from build123d import *
from build123d.topology import SkipClean

# Parameters (mm, degrees)
SKETCH1_W                = 100
SKETCH1_H                = 140
SKETCH1_R                = 2
EXTRUDE1_DEPTH           = 2
SKETCH2_W                = 60
SKETCH2_H                = 50
EXTRUDE2_DEPTH           = 87.046499057
SKETCH3_W                = 40
SKETCH3_H                = 20
EXTRUDE3_DEPTH           = 87.046499057
FILLET1_R                = 3
SKETCH4_W                = 6
SKETCH4_H                = 8
EXTRUDE4_DEPTH           = 60
SKETCH5_R                = 1
EXTRUDE5_DEPTH           = 8
SKETCH6_R                = 2
SKETCH6_R_2              = 2.1
EXTRUDE6_DEPTH           = 10
EXTRUDE_START            = -3
SKETCH_3_R               = 1.5
EXTRUDE_1_DEPTH          = 3
CUT_EXTRUDE_3_DEPTH      = 29
CUT_EXTRUDE_3_DEPTH_BACK = 134
SKETCH_4_W               = 103.957976386
SKETCH_4_H               = 74.150098407
SKETCH_6_R               = 2
CUT_EXTRUDE_4_DEPTH      = 11
SKETCH_8_R               = 2
CUT_EXTRUDE_6_DEPTH      = 11
EXTRUDE_START_2          = 1
SKETCH_9_R               = 2
SKETCH_9_R_2             = 2.1
EXTRUDE_2_DEPTH          = 1
SKETCH_10_R              = 1.6
CUT_EXTRUDE_7_DEPTH      = 3


with BuildPart() as part:
    # Sketch1 → Extrude1 (new body)
    with BuildSketch(Plane(origin=(0, 0, 0), x_dir=(1, 0, 0), z_dir=(0, 1, 0))):
        Rectangle(SKETCH1_W, SKETCH1_H)
        with Locations(Location((45, 65, 0), (0, 0, 270))):
            Circle(SKETCH1_R, mode=Mode.SUBTRACT)
        with Locations(Location((-45, 65, 0), (0, 0, 90))):
            Circle(SKETCH1_R, mode=Mode.SUBTRACT)
        with Locations(Location((-45, -65, 0), (0, 0, 270))):
            Circle(SKETCH1_R, mode=Mode.SUBTRACT)
        with Locations(Location((45, -65, 0), (0, 0, 90))):
            Circle(SKETCH1_R, mode=Mode.SUBTRACT)
    extrude(amount=EXTRUDE1_DEPTH)

    # Sketch2 → Extrude2 (cut, through all)
    with BuildSketch(Plane(origin=(0, 2, 0), x_dir=(1, 0, 0), z_dir=(0, 1, 0))):
        with Locations((0, -30)):
            Rectangle(SKETCH2_W, SKETCH2_H)
    extrude(amount=-EXTRUDE2_DEPTH, mode=Mode.SUBTRACT)

    # Sketch3 → Extrude3 (cut, through all)
    with BuildSketch(Plane(origin=(0, 2, 0), x_dir=(1, 0, 0), z_dir=(0, 1, 0))):
        with Locations((0, 30)):
            Rectangle(SKETCH3_W, SKETCH3_H)
    extrude(amount=-EXTRUDE3_DEPTH, mode=Mode.SUBTRACT)

    # Fillet1
    fillet1_edges = [part.edges().sort_by_distance(p)[0] for p in [
        (30, 1, 5),
        (30, 1, 55),
        (-30, 1, 55),
        (-30, 1, 5),
        (-20, 1, -20),
        (-20, 1, -40),
        (20, 1, -40),
        (20, 1, -20),
        (50, 1, 70),
        (-50, 1, 70),
        (-50, 1, -70),
        (50, 1, -70),
    ]]
    fillet(fillet1_edges, radius=FILLET1_R)

    # Sketch4 → Extrude4 (add)
    with BuildSketch(Plane.XZ):
        with Locations((47, 44)):
            Rectangle(SKETCH4_W, SKETCH4_H)
        with Locations((47, -24)):
            Rectangle(SKETCH4_W, SKETCH4_H)
        with Locations((-47, -24)):
            Rectangle(SKETCH4_W, SKETCH4_H)
        with Locations((-47, 44)):
            Rectangle(SKETCH4_W, SKETCH4_H)
    extrude(amount=EXTRUDE4_DEPTH)

    # Sketch5 → Extrude5 (add)
    # profile 1 of 4: a face of its own
    with BuildSketch(Plane.XZ.offset(60)):
        with BuildLine():
            Line((44, 40), (44, 48))
            Line((44, 48), (54, 48))
            ThreePointArc((54, 48), (58, 44), (54, 40))
            Line((54, 40), (44, 40))
        make_face()
        with Locations(Location((54, 44, 0), (0, 0, 270))):
            Circle(SKETCH5_R, mode=Mode.SUBTRACT)
    # profile 2 of 4: a face of its own
    with BuildSketch(Plane.XZ.offset(60)):
        with BuildLine():
            Line((44, -28), (44, -20))
            Line((44, -20), (54, -20))
            ThreePointArc((54, -20), (58, -24), (54, -28))
            Line((54, -28), (44, -28))
        make_face()
        with Locations(Location((54, -24, 0), (0, 0, 270))):
            Circle(SKETCH5_R, mode=Mode.SUBTRACT)
    # profile 3 of 4: a face of its own
    with BuildSketch(Plane.XZ.offset(60)):
        with BuildLine():
            Line((-44, -20), (-54, -20))
            ThreePointArc((-54, -20), (-58, -24), (-54, -28))
            Line((-54, -28), (-44, -28))
            Line((-44, -28), (-44, -20))
        make_face()
        with Locations(Location((-54, -24, 0), (0, 0, 90))):
            Circle(SKETCH5_R, mode=Mode.SUBTRACT)
    # profile 4 of 4: a face of its own
    with BuildSketch(Plane.XZ.offset(60)):
        with BuildLine():
            Line((-44, 48), (-54, 48))
            ThreePointArc((-54, 48), (-58, 44), (-54, 40))
            Line((-54, 40), (-44, 40))
            Line((-44, 40), (-44, 48))
        make_face()
        with Locations(Location((-54, 44, 0), (0, 0, 90))):
            Circle(SKETCH5_R, mode=Mode.SUBTRACT)
    extrude(amount=-EXTRUDE5_DEPTH)

    # Sketch6 → Extrude6 (cut)
    with BuildSketch(Plane(origin=(0, 0, 0), x_dir=(-1, 0, 0), z_dir=(0, -1, 0))):
        with Locations(Location((-47, -44, 0), (0, 0, 90))):
            Circle(SKETCH6_R)
        with Locations(Location((-47, 40, 0), (0, 0, 90))):
            Circle(SKETCH6_R_2)
        with Locations(Location((47, 40, 0), (0, 0, 270))):
            Circle(SKETCH6_R_2)
        with Locations(Location((47, -44, 0), (0, 0, 270))):
            Circle(SKETCH6_R)
    extrude(amount=-EXTRUDE6_DEPTH, mode=Mode.SUBTRACT)

    # Sketch 3 → Extrude 1 (add)
    # profile 1 of 4: a face of its own
    with BuildSketch(Plane(origin=(0, 2, 0), x_dir=(1, 0, 0), z_dir=(0, 1, 0)).offset(EXTRUDE_START)):
        with BuildLine():
            Line((50, 28), (50, 20))
            Line((50, 20), (54, 20))
            ThreePointArc((54, 20), (58, 24), (54, 28))
            Line((54, 28), (50, 28))
        make_face()
        with Locations(Location((54, 24, 0), (0, 0, 270))):
            Circle(SKETCH_3_R, mode=Mode.SUBTRACT)
    # profile 2 of 4: a face of its own
    with BuildSketch(Plane(origin=(0, 2, 0), x_dir=(1, 0, 0), z_dir=(0, 1, 0)).offset(EXTRUDE_START)):
        with BuildLine():
            Line((50, -40), (50, -48))
            Line((50, -48), (54, -48))
            ThreePointArc((54, -48), (58, -44), (54, -40))
            Line((54, -40), (50, -40))
        make_face()
        with Locations(Location((54, -44, 0), (0, 0, 270))):
            Circle(SKETCH_3_R, mode=Mode.SUBTRACT)
    # profile 3 of 4: a face of its own
    with BuildSketch(Plane(origin=(0, 2, 0), x_dir=(1, 0, 0), z_dir=(0, 1, 0)).offset(EXTRUDE_START)):
        with BuildLine():
            Line((-54, -48), (-50, -48))
            Line((-50, -48), (-50, -40))
            Line((-50, -40), (-54, -40))
            ThreePointArc((-54, -40), (-58, -44), (-54, -48))
        make_face()
        with Locations(Location((-54, -44, 0), (0, 0, 270))):
            Circle(SKETCH_3_R, mode=Mode.SUBTRACT)
    # profile 4 of 4: a face of its own
    with BuildSketch(Plane(origin=(0, 2, 0), x_dir=(1, 0, 0), z_dir=(0, 1, 0)).offset(EXTRUDE_START)):
        with BuildLine():
            Line((-50, 20), (-50, 28))
            Line((-50, 28), (-54, 28))
            ThreePointArc((-54, 28), (-58, 24), (-54, 20))
            Line((-54, 20), (-50, 20))
        make_face()
        with Locations(Location((-54, 24, 0), (0, 0, 270))):
            Circle(SKETCH_3_R, mode=Mode.SUBTRACT)
    extrude(amount=EXTRUDE_1_DEPTH)

    # Sketch 4 → Cut-Extrude 3 (cut, two sides: drawn at the far end of the back side and taken through both)
    with BuildSketch(Plane(origin=(50, 0, 0), x_dir=(0, 0, -1), z_dir=(1, 0, 0)).offset(-CUT_EXTRUDE_3_DEPTH_BACK)):
        with Locations((3.978988193, -38.075049204)):
            Rectangle(SKETCH_4_W, SKETCH_4_H)
    extrude(amount=CUT_EXTRUDE_3_DEPTH + CUT_EXTRUDE_3_DEPTH_BACK, mode=Mode.SUBTRACT)

    # Sketch 6 → Cut-Extrude 4 (cut)
    with BuildSketch(Plane(origin=(0, 2, 0), x_dir=(1, 0, 0), z_dir=(0, 1, 0))):
        with Locations(Location((-25, 60.55, 0), (0, 0, 270))):
            Circle(SKETCH_6_R)
        with Locations(Location((25, 60.55, 0), (0, 0, 270))):
            Circle(SKETCH_6_R)
    extrude(amount=-CUT_EXTRUDE_4_DEPTH, mode=Mode.SUBTRACT)

    # Sketch 8 → Cut-Extrude 6 (cut)
    with BuildSketch(Plane(origin=(0, 0, 0), x_dir=(-1, 0, 0), z_dir=(0, -1, 0))):
        with Locations(Location((25, -62.44, 0), (0, 0, 90))):
            Circle(SKETCH_8_R)
        with Locations(Location((-25, -62.44, 0), (0, 0, 270))):
            Circle(SKETCH_8_R)
    extrude(amount=-CUT_EXTRUDE_6_DEPTH, mode=Mode.SUBTRACT)

    # Sketch 9 → Extrude 2 (add)
    with BuildSketch(Plane.XZ.offset(EXTRUDE_START_2)):
        with BuildLine():
            Line((-44, 40), (-50, 40))
            Line((-50, 40), (-50, -20))
            Line((-50, -20), (-44, -20))
            Line((-44, -20), (-44, -28))
            Line((-44, -28), (-50, -28))
            Line((-50, -28), (-50, -67))
            ThreePointArc((-50, -67), (-49.121320344, -69.121320344), (-47, -70))
            Line((-47, -70), (47, -70))
            ThreePointArc((47, -70), (49.121320344, -69.121320344), (50, -67))
            Line((50, -67), (50, -28))
            Line((50, -28), (44, -28))
            Line((44, -28), (44, -20))
            Line((44, -20), (50, -20))
            Line((50, -20), (50, 40))
            Line((50, 40), (44, 40))
            Line((44, 40), (44, 48))
            Line((44, 48), (50, 48))
            Line((50, 48), (50, 67))
            ThreePointArc((50, 67), (49.121320344, 69.121320344), (47, 70))
            Line((47, 70), (-47, 70))
            ThreePointArc((-47, 70), (-49.121320344, 69.121320344), (-50, 67))
            Line((-50, 67), (-50, 48))
            Line((-50, 48), (-44, 48))
            Line((-44, 48), (-44, 40))
        make_face()
        with Locations(Location((-45, 65, 0), (0, 0, 270))):
            Circle(SKETCH_9_R, mode=Mode.SUBTRACT)
        with Locations(Location((-25, 62.44, 0), (0, 0, 270))):
            Circle(SKETCH_9_R, mode=Mode.SUBTRACT)
        with Locations(Location((45, 65, 0), (0, 0, 270))):
            Circle(SKETCH_9_R, mode=Mode.SUBTRACT)
        with Locations(Location((25, 62.44, 0), (0, 0, 270))):
            Circle(SKETCH_9_R, mode=Mode.SUBTRACT)
        with Locations(Location((47, -40, 0), (0, 0, 270))):
            Circle(SKETCH_9_R_2, mode=Mode.SUBTRACT)
        with Locations(Location((45, -65, 0), (0, 0, 270))):
            Circle(SKETCH_9_R, mode=Mode.SUBTRACT)
        with Locations(Location((25, -60.55, 0), (0, 0, 270))):
            Circle(SKETCH_9_R, mode=Mode.SUBTRACT)
        with Locations(Location((-45, -65, 0), (0, 0, 270))):
            Circle(SKETCH_9_R, mode=Mode.SUBTRACT)
        with Locations(Location((-47, -40, 0), (0, 0, 270))):
            Circle(SKETCH_9_R_2, mode=Mode.SUBTRACT)
        with Locations(Location((-25, -60.55, 0), (0, 0, 90))):
            Circle(SKETCH_9_R, mode=Mode.SUBTRACT)
        with BuildLine():
            Line((30, 52), (30, 8))
            ThreePointArc((30, 8), (29.121320344, 5.878679656), (27, 5))
            Line((27, 5), (-27, 5))
            ThreePointArc((-27, 5), (-29.121320344, 5.878679656), (-30, 8))
            Line((-30, 8), (-30, 52))
            ThreePointArc((-30, 52), (-29.121320344, 54.121320344), (-27, 55))
            Line((-27, 55), (27, 55))
            ThreePointArc((27, 55), (29.121320344, 54.121320344), (30, 52))
        make_face(mode=Mode.SUBTRACT)
        with BuildLine():
            Line((20, -23), (20, -37))
            ThreePointArc((20, -37), (19.121320344, -39.121320344), (17, -40))
            Line((17, -40), (-17, -40))
            ThreePointArc((-17, -40), (-19.121320344, -39.121320344), (-20, -37))
            Line((-20, -37), (-20, -23))
            ThreePointArc((-20, -23), (-19.121320344, -20.878679656), (-17, -20))
            Line((-17, -20), (17, -20))
            ThreePointArc((17, -20), (19.121320344, -20.878679656), (20, -23))
        make_face(mode=Mode.SUBTRACT)
    extrude(amount=-EXTRUDE_2_DEPTH)

    # Sketch 10 → Cut-Extrude 7 (cut)
    with SkipClean():  # the faces are left unmerged after this step: merging them gives an invalid solid
        with BuildSketch(Plane(origin=(0, -1, 0), x_dir=(-1, 0, 0), z_dir=(0, -1, 0))):
            with Locations(Location((34.25, 6.5, 0), (0, 0, 90))):
                Circle(SKETCH_10_R)
            with Locations(Location((-34.25, 6.5, 0), (0, 0, 270))):
                Circle(SKETCH_10_R)
        extrude(amount=-CUT_EXTRUDE_7_DEPTH, mode=Mode.SUBTRACT)
    add(part.part.scale(1), mode=Mode.REPLACE)  # the faces are merged on a copy


solid = part.part
Here's how the part is built. I have some questions about the finished solid (model axes, mm). A direction names the side the tool comes from. Give positions to 0.01 mm unless a question says otherwise; leave off trailing zeros. Order: outer loops, then holes, each group sorted by start corner. A loop starts at its lowest first (then second) coordinate and runs counter-clockwise, first axis right, second up. Notation, with made-up numbers: M -21,-27.75 L 13,-27.75 A21 ccw 13,-4.75 Z; hole C 67,-37.75 d10. An arc over 180 degrees is marked long. Answer as a JSON object with one key per item and string values. Group by question number.
1) Suppose I cut it at B-B, the plane z = 11.5. Write out the boundary of the cut face in (x, y).
2) We'd pull the mould along Z, two halves only. Please class faces 1 (the flat face through (50, 0, -48)), 2 (the cylindrical face through (-54.9, 0.5, 42.8)), 3 (the flat face through (-50, 0, 10)), 4 (the flat face through (1, 0, 70)): pulls with the +Z half, pulls with the -Z half, needs draft (parallel to the pull), parting line crosses it, or undercut.
3) Please list where these lines run through material, in increasing order: L1, parallel to X at y = 0.85, z = -60.55; L2, parallel to X at y = 1.45, z = 44; L3, parallel to Z at x = -6.5, y = 0.25. Write a range as [from, to].
4) Suppose I cut it at A-A, the plane x = 34.25. Write out the boundary of the cut face in (y, z), plus the area to 3 significant figures.
5) Suppose I cut it at C-C, the plane z = 44. Write out the boundary of the cut face in (x, y).
6) Suppose I cut it at D-D, the plane x = -25. Write out the boundary of the cut face in (y, z).
7) On a 3-axis mill with a long thin cutter (end or side, diameter ignored), from which of +Z, -Z, +X, -X, +Y, -Y can I reach the whole of each face in a straight line? I mean faces 5 (the cylindrical face through (45, 1, 44)), 6 (the flat face through (52, 0, -20)), 7 (the flat face through (-50, 0, -47)), 8 (the flat face through (50, 0, 57)). Say none if no direction works.
8) I'm going to push flat-ended pins straight in: pin 1 Ø2 at (x, z) = (24, 53.5) entering from -Y (3 decimals); pin 2 Ø1.1 at (y, z) = (-0.5, 26.5) entering from +X; pin 3 Ø0.9 at (x, y) = (52.5, 0.5) entering from +Z; pin 4 Ø1 at (y, z) = (1.5, -53.5) entering from -X. Where does each tip first touch, or does it pass through?
Results found:
{
 "1": {"outline": "M -50,-1 L -30,-1 L -30,2 L -50,2 Z; M 30,-1 L 50,-1 L 50,2 L 30,2 Z"},
 "2": {"face 1": "needs draft", "face 2": "undercut", "face 3": "undercut", "face 4": "pulls with the +Z half"},
 "3": {"L1": "[-50, -27], [-23, 23], [27, 50]", "L2": "[-58, -55.5], [-52.5, -49], [-45, -30], [30, 45], [49, 52.5], [55.5, 58]", "L3": "[-70, -40], [-20, 5], [55, 70]"},
 "4": {"outline": "M -1,-70 L 2,-70 L 2,-8.1 L -1,-8.1 Z; M -1,-4.9 L 2,-4.9 L 2,70 L -1,70 Z", "area": "410 mm²"},
 "5": {"outline": "M -58,-1 L -55.5,-1 L -55.5,2 L -58,2 Z; M -52.5,-1 L -30,-1 L -30,2 L -45,2 L -45,0 L -49,0 L -49,2 L -52.5,2 Z; M 30,-1 L 52.5,-1 L 52.5,2 L 49,2 L 49,0 L 45,0 L 45,2 L 30,2 Z; M 55.5,-1 L 58,-1 L 58,2 L 55.5,2 Z"},
 "6": {"outline": "M -1,-70 L 2,-70 L 2,-62.55 L -1,-62.55 Z; M -1,-58.55 L 2,-58.55 L 2,5 L -1,5 Z; M -1,55 L 2,55 L 2,60.44 L -1,60.44 Z; M -1,64.44 L 2,64.44 L 2,70 L -1,70 Z"},
 "7": {"face 5": "+Y", "face 6": "+X, +Y, -Y", "face 7": "-Z, -X, +Y, -Y", "face 8": "+Z, +X, +Y, -Y"},
 "8": {"pin 1": "through", "pin 2": "x = 50", "pin 3": "z = 48", "pin 4": "x = -50"}
}
